Can you work these out from the model? Positions are in its coordinate system, mm. A direction names the side the tool comes from. Round coordinates to 2 decimals unless told otherwise and drop trailing zeros. Loops run counter-clockwise (first coordinate to the right, second up) from the corner with the lowest first, then second, coordinate; pieces in that order, holes last.
(1) Thinking about a two-plate mould opening in Y: for faces 1 (the face through (2, 47.625, 51)), 2 (the face through (1.61, -41.72, -46.98)), 3 (the face through (2, 49, 12.7)), 4 (the face through (2, 0, -62)), which applies, released by +Y, released by -Y, zero draft, split by the parting line, or undercut?
(2) Which directions (+Z, -Z, +X, -X, +Y, -Y) give clear straight access to the entire face, cutting with the end or side of a thin tool? Please do faces 5 (the face through (2, 13, 60.325)), 6 (the face through (2, -34.925, 25)), 7 (the face through (2, 47.625, -51)).
(3) If I drill on line 1 along Y through (x, z) = (2.05, 0); line 2 along Y through (x, z) = (0.3, -3) (3 decimals); line 3 along Z through (x, y) = (2.25, -17), over which ranges is the centre line in solid material (lowest first)?
(4) I want a section at A-A on y = -21. Write out the boundary of the cut face in (x, z) (3 decimals).
(5) I want a section at C-C on z = 0. Write out the boundary of the cut face in (x, y) (3 decimals), plus the area to 3 significant figures.
(6) I want a section at D-D on x = 1.75. Give the number of separate pieces and of enclosed holes in the cut face, plus the area to 3 significant figures.
(7) I want a section at B-B on z = 33. Write out the boundary of the cut face in (x, y) (3 decimals).
(8) Will these pins go through, and if not, where does the flat tip stop? pin 1 Ø1 at (x, z) = (1, -45) entering from -Y; pin 2 Ø1 at (x, y) = (2, 16) entering from -Z (3 decimals); pin 3 Ø1.8 at (x, z) = (2, -3) entering from +Y (3 decimals).
from build123d import *

# Parameters (mm, degrees)
SKETCH1_W                 = 127
SKETCH1_H                 = 101.6
BOSS_EXTRUDE1_DEPTH       = 3.175
SKETCH2_W                 = 25.4
SKETCH2_H                 = 3.175
CUT_EXTRUDE1_DEPTH        = 6.35
LPATTERN1_COUNT           = 3
LPATTERN1_PITCH           = 50.8
CUT_EXTRUDE4_DEPTH        = 6.35
SKETCH8_W                 = 3.175
SKETCH8_H                 = 25.4
CUT_EXTRUDE6_DEPTH        = 6.35
SKETCH9_W                 = 25.4
SKETCH9_H                 = 3.175
CUT_EXTRUDE7_DEPTH        = 6.35
LPATTERN6_COUNT           = 2
LPATTERN6_PITCH           = 50.8
SKETCH16_W                = 4.3942
SKETCH16_H                = 17.145
SKETCH16_W_2              = 8.89
SKETCH16_H_2              = 3.302
CUT_EXTRUDE14_DEPTH       = 6.35
F_8_CLEARANCE_HOLE1_D     = 4.4958
F_8_CLEARANCE_HOLE1_DEPTH = 10.16
F_8_CLEARANCE_HOLE1_TIP   = 1.350674586
SKETCH20_R                = 1.143
SKETCH20_W                = 23.622
SKETCH20_H                = 23.622
CUT_EXTRUDE16_DEPTH       = 10.16


with BuildPart() as part:
    # Sketch1 → Boss-Extrude1 (new body)
    with BuildSketch(Plane(origin=(0, 0, 0), x_dir=(0, 0, -1), z_dir=(1, 0, 0))):
        Rectangle(SKETCH1_W, SKETCH1_H)
    extrude(amount=BOSS_EXTRUDE1_DEPTH)

    # Sketch2 → Cut-Extrude1 (cut)
    with BuildSketch(Plane(origin=(3.175, 0, 0), x_dir=(0, 0, -1), z_dir=(1, 0, 0))):
        with Locations((-50.8, 49.2125)):
            Rectangle(SKETCH2_W, SKETCH2_H)
    cut_extrude1 = extrude(amount=-CUT_EXTRUDE1_DEPTH, mode=Mode.SUBTRACT)

    # LPattern1: Cut-Extrude1 ×3
    with Locations(*[(0, 0, -i * LPATTERN1_PITCH) for i in range(1, LPATTERN1_COUNT)]):
        add(cut_extrude1, mode=Mode.SUBTRACT)

    # Sketch5 → Cut-Extrude4 (cut)
    with BuildSketch(Plane(origin=(3.175, 0, 0), x_dir=(0, 0, -1), z_dir=(1, 0, 0))):
        with BuildLine():
            Line((-38.1, -38.1), (38.1, -38.1))
            ThreePointArc((38.1, -38.1), (50.8, -50.8), (38.1, -63.5))
            Line((38.1, -63.5), (-38.1, -63.5))
            ThreePointArc((-38.1, -63.5), (-50.8, -50.8), (-38.1, -38.1))
        make_face()
    extrude(amount=-CUT_EXTRUDE4_DEPTH, mode=Mode.SUBTRACT)

    # Sketch8 → Cut-Extrude6 (cut)
    with BuildSketch(Plane(origin=(3.175, 0, 0), x_dir=(0, 0, -1), z_dir=(1, 0, 0))):
        with Locations((61.9125, 12.7)):
            Rectangle(SKETCH8_W, SKETCH8_H)
    cut_extrude6 = extrude(amount=-CUT_EXTRUDE6_DEPTH, mode=Mode.SUBTRACT)

    # Sketch9 → Cut-Extrude7 (cut)
    with BuildSketch(Plane.ZY):
        with Locations((-25.4, -33.3375)):
            Rectangle(SKETCH9_W, SKETCH9_H)
    cut_extrude7 = extrude(amount=-CUT_EXTRUDE7_DEPTH, mode=Mode.SUBTRACT)

    # LPattern6: Cut-Extrude7 ×2
    with Locations(*[(0, 0, i * LPATTERN6_PITCH) for i in range(1, LPATTERN6_COUNT)]):
        add(cut_extrude7, mode=Mode.SUBTRACT)

    # Sketch16 → Cut-Extrude14 (cut)
    with BuildSketch(Plane.ZY):
        with Locations((0, 39.0525)):
            Rectangle(SKETCH16_W, SKETCH16_H)
        with Locations((0, 41.275)):
            Rectangle(SKETCH16_W_2, SKETCH16_H_2)
    extrude(amount=-CUT_EXTRUDE14_DEPTH, mode=Mode.SUBTRACT)

    # #8 Clearance Hole1
    with Locations(Plane.ZY):
        with Locations((0, -33.3375)):
            Hole(F_8_CLEARANCE_HOLE1_D / 2, depth=F_8_CLEARANCE_HOLE1_DEPTH)
            with Locations((0, 0, -(F_8_CLEARANCE_HOLE1_DEPTH + F_8_CLEARANCE_HOLE1_TIP / 2))):  # 118° drill point
                Cone(0, F_8_CLEARANCE_HOLE1_D / 2, F_8_CLEARANCE_HOLE1_TIP, mode=Mode.SUBTRACT)

    # Sketch20 → Cut-Extrude16 (cut)
    with BuildSketch(Plane.ZY):
        with Locations((-14.986, -13.589)):
            Circle(SKETCH20_R)
        with Locations((14.986, -13.589)):
            Circle(SKETCH20_R)
        with Locations((0, -13.589)):
            Rectangle(SKETCH20_W, SKETCH20_H)
    extrude(amount=-CUT_EXTRUDE16_DEPTH, mode=Mode.SUBTRACT)

    # Mirror3: Cut-Extrude6 across plane
    add(cut_extrude6.mirror(Plane.XY), mode=Mode.SUBTRACT)


solid = part.part
Filled sheet:
1. face 1: released by +Y
1. face 2: released by -Y
1. face 3: zero draft
1. face 4: undercut
2. face 5: +Z, +X, -X
2. face 6: +X, -X
2. face 7: -Z, +X, -X, +Y
3. line 1: y = -38.1 to -35.59, -31.09 to -25.4, -1.78 to 30.48
3. line 2: y = -38.1 to -25.4, -1.778 to 39.624, 42.926 to 47.625
3. line 3: z = -63.5 to -11.81, 11.81 to 63.5
4. outline: (0, -63.5) - (3.175, -63.5) - (3.175, -11.811) - (0, -11.811) - close; (0, 11.811) - (3.175, 11.811) - (3.175, 63.5) - (0, 63.5) - close
5. outline: (0, -38.1) - (3.175, -38.1) - (3.175, -35.585) - (0, -35.585) - close; (0, -31.09) - (3.175, -31.09) - (3.175, -25.4) - (0, -25.4) - close; (0, -1.778) - (3.175, -1.778) - (3.175, 30.48) - (0, 30.48) - close
5. area: 128 mm2
6. separate pieces: 1
6. enclosed holes: 6
6. area: 10,400 mm2
7. outline: (0, -38.1) - (3.175, -38.1) - (3.175, -34.925) - (0, -34.925) - close; (0, -31.75) - (3.175, -31.75) - (3.175, 50.8) - (0, 50.8) - close
8. pin 1: stops at y = -40.48
8. pin 2: stops at z = -60.325
8. pin 3: stops at y = 47.625
